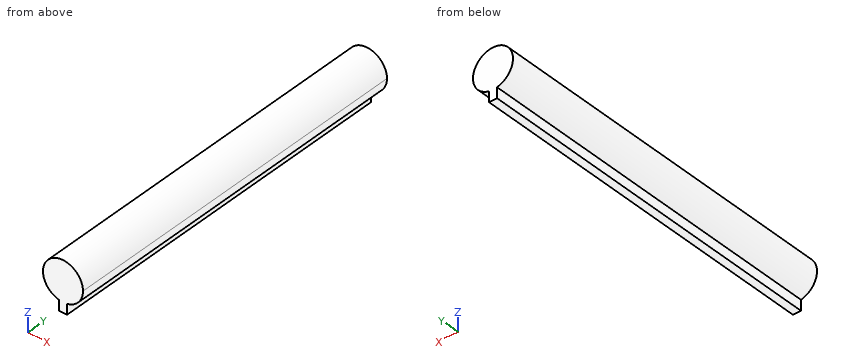
```python
from build123d import *

# Parameters (mm, degrees)
SKETCH1_R           = 2
BOSS_EXTRUDE1_DEPTH = 45
CUT_EXTRUDE1_START  = -53
SKETCH2_R           = 4.181773236
CUT_EXTRUDE1_DEPTH  = 53
SKETCH3_R           = 2.328270144
CUT_EXTRUDE2_DEPTH  = 27


with BuildPart() as part:
    # Sketch1 → Boss-Extrude1 (new body)
    with BuildSketch(Plane(origin=(0, 0, 0), x_dir=(1, 0, 0), z_dir=(0, 1, 0))):
        Polygon((-0.5, 1.936491673), (0, 2.368245837), (0, 2.8), (-0.5, 2.8), align=None)
        Polygon((0, 2.8), (0, 2.368245837), (0.5, 2.8), align=None)
        with BuildLine():
            Line((0, 2.368245837), (0, 2))
            ThreePointArc((0, 2), (0.252008585, 1.984059393), (0.5, 1.936491673))
            Line((0.5, 1.936491673), (0.5, 2.8))
            Line((0.5, 2.8), (0, 2.368245837))
        make_face()
        with BuildLine():
            ThreePointArc((-0.5, 1.936491673), (-0.252008585, 1.984059393), (0, 2))
            Line((0, 2), (0, 2.368245837))
            Line((0, 2.368245837), (-0.5, 1.936491673))
        make_face()
        Circle(SKETCH1_R)
    extrude(amount=BOSS_EXTRUDE1_DEPTH)

    # Sketch2 → Cut-Extrude1 (cut)
    # profile 1 of 2: a face of its own
    with BuildSketch(Plane(origin=(0, 45, 0), x_dir=(1, 0, 0), z_dir=(0, 1, 0)).offset(CUT_EXTRUDE1_START)):
        Circle(SKETCH2_R)
        with BuildLine():
            Line((-0.5, 2.8), (-0.5, 1.936491673))
            ThreePointArc((-0.5, 1.936491673), (0, -2), (0.5, 1.936491673))
            Line((0.5, 1.936491673), (0.5, 2.8))
            Line((0.5, 2.8), (-0.5, 2.8))
        make_face(mode=Mode.SUBTRACT)
    # profile 2 of 2: a face of its own
    with BuildSketch(Plane(origin=(0, 45, 0), x_dir=(1, 0, 0), z_dir=(0, 1, 0)).offset(CUT_EXTRUDE1_START)):
        with BuildLine():
            Line((0.5, 2.8), (-0.5, 2.8))
            Line((-0.5, 2.8), (-0.5, 1.936491673))
            ThreePointArc((-0.5, 1.936491673), (0, -2), (0.5, 1.936491673))
            Line((0.5, 1.936491673), (0.5, 2.8))
        make_face()
        with BuildLine():
            Line((-0.20151518, 1.5), (0, 1.5))
            Line((0, 1.5), (0.2, 1.5))
            Line((0.2, 1.5), (0.2, 0.979795897))
            ThreePointArc((0.2, 0.979795897), (0.774596669, 0.632455532), (1, 0))
            ThreePointArc((1, 0), (-0.631856321, -0.775085537), (-0.20151518, 0.979485391))
            Line((-0.20151518, 0.979485391), (-0.20151518, 1.5))
        make_face(mode=Mode.SUBTRACT)
    extrude(amount=CUT_EXTRUDE1_DEPTH, mode=Mode.SUBTRACT)

    # Sketch3 → Cut-Extrude2 (cut)
    with BuildSketch(Plane(origin=(0, 45, 0), x_dir=(1, 0, 0), z_dir=(0, 1, 0))):
        Circle(SKETCH3_R)
    extrude(amount=-CUT_EXTRUDE2_DEPTH, mode=Mode.SUBTRACT)


solid = part.part
```
Geometry: final body of the model. Coordinates: model frame, mm. Round coordinates to 2 decimals unless told otherwise and drop trailing zeros. Loops run counter-clockwise (first coordinate to the right, second up) from the corner with the lowest first, then second, coordinate; pieces in that order, holes last.
Item 1: Section A-A, the plane y = 14.75. Output: boundary loops of the cut face in (x, z), plus the area to 3 significant figures.
Checked values:
outline: (-0.2, -1.5) - (0.2, -1.5) - (0.2, -0.98) arc R1 ccw (long way) to (-0.2, -0.98) - close
area: 3.35 mm2
Item 2: Section B-B, the plane z = -0.8. Output: boundary loops of the cut face in (x, y).
Checked values:
outline: (-0.6, 0) - (0.6, 0) - (0.6, 18) - (-0.6, 18) - close
Item 3: Contact query for a flat-ended pin moving along its axis: P1, Ø1, axis at x = 1, y = 14, coming from the +Z side. Output: stop coordinate, or through.
Checked values:
P1: stops at z = 0.87
Item 4: Line query: L1, parallel to X at y = 11, z = 0.05; L2, parallel to X at y = 12.25, z = -1.35; L3, parallel to Z at x = -0.55, y = 6.25. Output: solid intervals per line, ascending.
Checked values:
L1: x = -1 to 1
L2: x = -0.2 to 0.2
L3: z = -0.84 to 0.84
Item 5: Section C-C, the plane x = 0.6. Output: boundary loops of the cut face in (y, z), plus the area to 3 significant figures.
Checked values:
outline: (0, -0.8) - (18, -0.8) - (18, 0.8) - (0, 0.8) - close
area: 28.8 mm2
